Read the model definition and answer for the solid it produces. Units are mm, in the model's axes. A direction names the side the tool comes from. Round coordinates to 2 decimals unless told otherwise and drop trailing zeros. Order: outer loops, then holes, each group sorted by start corner. A loop starts at its lowest first (then second) coordinate and runs counter-clockwise, first axis right, second up.
from build123d import *

# Parameters (mm, degrees)
SKETCH_1_R          = 23
SKETCH_1_R_2        = 1.5
SKETCH_1_R_3        = 11.1
EXTRUDE_1_DEPTH     = 1.5
CUT_EXTRUDE_1_DEPTH = 2.5


with BuildPart() as part:
    # 草图1 → 凸台-拉伸1 (new body)
    with BuildSketch(Plane.XY):
        Circle(SKETCH_1_R)
        with Locations((0, 20)):
            Circle(SKETCH_1_R_2, mode=Mode.SUBTRACT)
        Circle(SKETCH_1_R_3, mode=Mode.SUBTRACT)
        with Locations((17.320508076, -10)):
            Circle(SKETCH_1_R_2, mode=Mode.SUBTRACT)
        with Locations((-17.320508076, -10)):
            Circle(SKETCH_1_R_2, mode=Mode.SUBTRACT)
    extrude(amount=EXTRUDE_1_DEPTH)

    # 草图2 → 切除-拉伸1 (cut, through all)
    with BuildSketch(Plane.XY.offset(1.5)):
        with BuildLine():
            ThreePointArc((-8.452365235, 18.126155741), (-17.320508076, 10), (-19.923893962, -1.743114855))
            ThreePointArc((-19.923893962, -1.743114855), (-16.728010161, -4.424779773), (-14.046345243, -1.228895973))
            ThreePointArc((-14.046345243, -1.228895973), (-12.210958193, 7.05), (-5.958917491, 12.778939797))
            ThreePointArc((-5.958917491, 12.778939797), (-4.532033391, 16.699271641), (-8.452365235, 18.126155741))
        make_face()
        with BuildLine():
            ThreePointArc((19.923893962, -1.743114855), (17.320508076, 10), (8.452365235, 18.126155741))
            ThreePointArc((8.452365235, 18.126155741), (4.532033391, 16.699271641), (5.958917491, 12.778939797))
            ThreePointArc((5.958917491, 12.778939797), (12.210958193, 7.05), (14.046345243, -1.228895973))
            ThreePointArc((14.046345243, -1.228895973), (16.728010161, -4.424779773), (19.923893962, -1.743114855))
        make_face()
        with BuildLine():
            ThreePointArc((-11.471528727, -16.383040886), (0, -20), (11.471528727, -16.383040886))
            ThreePointArc((11.471528727, -16.383040886), (12.19597677, -12.274491868), (8.087427753, -11.550043824))
            ThreePointArc((8.087427753, -11.550043824), (0, -14.1), (-8.087427753, -11.550043824))
            ThreePointArc((-8.087427753, -11.550043824), (-12.19597677, -12.274491868), (-11.471528727, -16.383040886))
        make_face()
    extrude(amount=-CUT_EXTRUDE_1_DEPTH, mode=Mode.SUBTRACT)


solid = part.part
Q1. A flat-ended cylindrical pin translates along its axis: pin 1 (8 mm diameter, centred on x = 6.5, y = 14.5, fed in from +Z). Find the tip coordinate at first contact, or state that the pin passes through.
Outcome:
pin 1: stops at z = 1.5
Q2. For faces 4 (the face through (0, -20, 1)), 5 (the face through (-5.4, -9.9, 1.5)), determine the directions among +Z, -Z, +X, -X, +Y, -Y from which every point of the face is accessible in a straight line to the end or side of a thin tool.
Outcome:
face 4: +Z, -Z
face 5: +Z, +X, -X, +Y, -Y
Q3. A cutting plane is placed at B-B, the plane y = 0. Give the vertices of the cut face in (x, z), plus the area to 3 significant figures.
Outcome:
outline: (-23, 0) - (-20, 0) - (-20, 1.5) - (-23, 1.5) - close; (-14.1, 0) - (-11.1, 0) - (-11.1, 1.5) - (-14.1, 1.5) - close; (11.1, 0) - (14.1, 0) - (14.1, 1.5) - (11.1, 1.5) - close; (20, 0) - (23, 0) - (23, 1.5) - (20, 1.5) - close
area: 18.0 mm2
Q4. For a pull along X with two mould halves and no side action, classify faces 1 (the face through (-2.994, 22.804, 0.74)), 2 (the face through (-12.158, -12.222, 0.76)), 3 (the face through (-5.4, -9.9, 0)) as released by +X, released by -X, zero draft, split by the parting line, or undercut.
Outcome:
face 1: split by the parting line
face 2: undercut
face 3: zero draft
Q5. Straight lines are drawn through the part: probe 1 along Y at (x, z) = (0, 0.7); probe 2 along X at (y, z) = (13, 1.45); probe 3 along X at (y, z) = (10, 1.1). For each, find the intervals that lie inside material, in ascending order.
Outcome:
probe 1: y = -23 to -20, -14.1 to -11.1, 11.1 to 18.5, 21.5 to 23
probe 2: x = -18.97 to -15.2, -5.57 to 5.57, 15.2 to 18.97
probe 3: x = -20.71 to -17.32, -9.94 to -4.82, 4.82 to 9.94, 17.32 to 20.71
Q6. A cutting plane is placed at D-D, the plane z = 0.5. Give the vertices of the cut face in (x, y).
Outcome:
outline: circle Ø46 at (0, 0); hole (-19.92, -1.74) arc R2.95 ccw to (-14.05, -1.23) arc R14.1 cw to (-5.96, 12.78) arc R2.95 ccw to (-8.45, 18.13) arc R20 ccw to start; hole circle Ø3 at (-17.32, -10); hole (-11.47, -16.38) arc R20 ccw to (11.47, -16.38) arc R2.95 ccw to (8.09, -11.55) arc R14.1 cw to (-8.09, -11.55) arc R2.95 ccw to start; hole circle Ø22.2 at (0, 0); hole circle Ø3 at (0, 20); hole (5.96, 12.78) arc R14.1 cw to (14.05, -1.23) arc R2.95 ccw to (19.92, -1.74) arc R20 ccw to (8.45, 18.13) arc R2.95 ccw to start; hole circle Ø3 at (17.32, -10)
Q7. A cutting plane is placed at C-C, the plane y = 20. Give the vertices of the cut face in (x, z).
Outcome:
outline: (-11.36, 0) - (-1.5, 0) - (-1.5, 1.5) - (-11.36, 1.5) - close; (1.5, 0) - (11.36, 0) - (11.36, 1.5) - (1.5, 1.5) - close
Q8. A cutting plane is placed at A-A, the plane x = 0. Give the vertices of the cut face in (y, z), plus the area to 4 significant figures.
Outcome:
outline: (-23, 0) - (-20, 0) - (-20, 1.5) - (-23, 1.5) - close; (-14.1, 0) - (-11.1, 0) - (-11.1, 1.5) - (-14.1, 1.5) - close; (11.1, 0) - (18.5, 0) - (18.5, 1.5) - (11.1, 1.5) - close; (21.5, 0) - (23, 0) - (23, 1.5) - (21.5, 1.5) - close
area: 22.35 mm2
